from build123d import *

# Parameters (mm, degrees)
F0_W     = 60
F0_H     = 60
F1_DEPTH = 330
F3_DEPTH = 40
F4_W     = 5
F4_H     = 19
F5_DEPTH = 15
F6_W     = 5
F6_H     = 19
F7_DEPTH = 15


with BuildPart() as f1:
    # F0 (on Top) → F1 (new body)
    with BuildSketch(Plane.XY):
        Rectangle(F0_W, F0_H)
    extrude(amount=-F1_DEPTH)

    # F2 (on face) → F3 (cut)
    with BuildSketch(Plane.XY):
        Polygon((30, 30), (-1, 30), (30, -1), align=None)
    extrude(amount=-F3_DEPTH, mode=Mode.SUBTRACT)

    # F4 (on face) → F5 (cut)
    with BuildSketch(Plane.YZ.offset(30)):
        with Locations((-10, -16.5)):
            Rectangle(F4_W, F4_H)
        with Locations((-10, -43.5)):
            Rectangle(F4_W, F4_H)
    extrude(amount=-F5_DEPTH, mode=Mode.SUBTRACT)

    # F6 (on face) → F7 (cut)
    with BuildSketch(Plane(origin=(0, 30, 0), x_dir=(-1, 0, 0), z_dir=(0, 1, 0))):
        with Locations((10, -16.5)):
            Rectangle(F6_W, F6_H)
        with Locations((10, -43.5)):
            Rectangle(F6_W, F6_H)
    extrude(amount=-F7_DEPTH, mode=Mode.SUBTRACT)


solid = f1.part
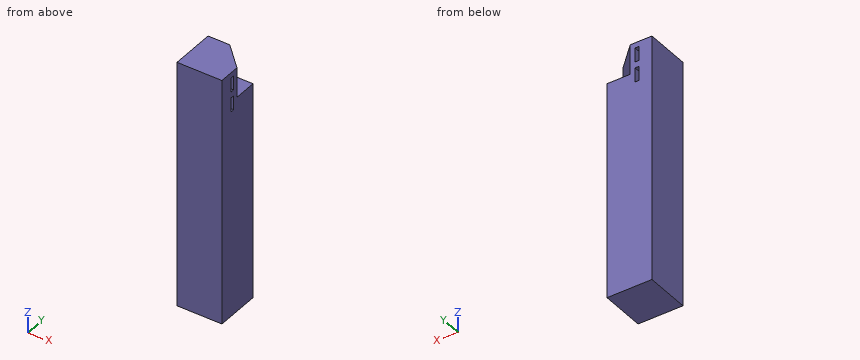
The listing builds one solid part. Answer for the finished solid, in the listing's coordinates (mm). Coordinates: 2 decimals unless noted, no trailing zeros. Write each loop counter-clockwise with the first axis right and the second up, starting at its lowest first coordinate (ties: lowest second). Pieces come first, ordered by that corner, then holes. Notation, with made-up numbers: M -9.75,-20.5 L 43.25,-20.5 A20 cw 43.25,10.5 Z; hole C 72.5,11 d5. An arc over 180 degrees is marked long. Put each result on its own line as item: value. Start each with the question number.
1. A cutting plane is placed at C-C on y = 8. Write down the section's boundary in (x, z).
2. A cutting plane is placed at B-B on z = -21. Write down the section's boundary in (x, y).
3. Consider line 1 (X direction, y = -12, z = -38); line 2 (Z direction, x = 10.5, y = 25); line 3 (X direction, y = 3.5, z = -20). Determine where each line is inside the solid, lowest interval first. Write a range as from..to.
4. A cutting plane is placed at A-A on x = 26.5. Write down the section's boundary in (y, z), then the cut area to 3 significant figures.
5. Flat-ended cylindrical pins translate along their axes: P1, Ø4, axis at x = 26, y = -10.5, coming from the +Z side; P2, Ø4.5, axis at x = 19.5, z = -19.5, coming from the +Y side. Find the tip coordinate at first contact, or state that the pin passes through.
Resolved:
1. outline: M -30,-330 L 30,-330 L 30,-40 L 21,-40 L 21,0 L -30,0 Z
2. outline: M -30,-30 L 30,-30 L 30,-12.5 L 15,-12.5 L 15,-7.5 L 30,-7.5 L 30,-1 L -1,30 L -7.5,30 L -7.5,15 L -12.5,15 L -12.5,30 L -30,30 Z
3. line 1: x = -30..15
3. line 2: z = -330..-40
3. line 3: x = -30..25.5
4. outline: M -30,-330 L 30,-330 L 30,-40 L 2.5,-40 L 2.5,0 L -30,0 Z; hole M -12.5,-53 L -7.5,-53 L -7.5,-34 L -12.5,-34 Z; hole M -12.5,-26 L -7.5,-26 L -7.5,-7 L -12.5,-7 Z
4. area: 18,500 mm2
5. P1: stops at z = 0
5. P2: stops at y = 11.75
